Here's how the part is built. I have some questions about the finished solid (model axes, mm). A direction names the side the tool comes from. Give positions to 0.01 mm unless a question says otherwise; leave off trailing zeros. Write each loop counter-clockwise with the first axis right and the second up, starting at its lowest first coordinate (ties: lowest second). Pieces come first, ordered by that corner, then holes. Notation, with made-up numbers: (6, 82) - (64, 82) arc R9 cw to (64, 93) - close; hole circle Ø6 at (-13.75, 88). An arc over 180 degrees is marked (long way). Write each question's results on one line, items separated by ' | '. Start each with the question number.
Item 1: Please list where these lines run through material, in increasing order: line 1 along X through (y, z) = (1.5, 12); line 2 along Y through (x, z) = (2, 0); line 3 along Z through (x, y) = (34, 11.25).
Item 2: Suppose I cut it at B-B on z = 27. List the corners of the cut face in (x, y) for me.
Item 3: Suppose I cut it at A-A on y = 8.55. List the corners of the cut face in (x, z) for me, then the cut area to 3 significant figures.
Item 4: Suppose I cut it at C-C on x = -0.5. List the corners of the cut face in (y, z) for me, then the cut area to 3 significant figures.
Item 5: We'd pull the mould along X, two halves only. Please class faces 1 (the flat face through (20, 8, 33.821)), 2 (the cylindrical face through (31.889, 17.646, 28.891)), 3 (the cylindrical face through (33.25, 10.43, 28.89)): +X half, -X half, draft (parallel to the pull), parting line (faces both ways), or undercut.
Item 6: Which directions (+Z, -Z, +X, -X, +Y, -Y) give clear straight access to the entire face, cutting with the end or side of a thin tool? Please do faces 4 (the flat face through (19.209, 1, 10)), 5 (the cylindrical face through (16.13, 4.3, 28.89)), 6 (the flat face through (9, 1, -4.379)), 7 (the flat face through (7, 3, 14)), 8 (the flat face through (-3.991, 1, 15)).
Item 7: Suppose I cut it at D-D on x = 16. List the corners of the cut face in (y, z) for me.
Item 8: Will these pins go through, and if not, where does the flat tip stop? P1, Ø3.5, axis at x = 6.21, z = 29.82, coming from the +Y side; P2, Ø8, axis at y = 3.5, z = 0.5, coming from the +X side.
```python
from build123d import *

# Parameters (mm, degrees)
SKETCH1_W           = 23.2
SKETCH1_H           = 38.2
SKETCH1_R           = 1.6
BOSS_EXTRUDE1_DEPTH = 3
FILLET1_R           = 4
SKETCH2_R           = 6.25
BOSS_EXTRUDE2_DEPTH = 10
FILLET2_R           = 4


with BuildPart() as part:
    # Sketch1 → Boss-Extrude1 (new body)
    with BuildSketch(Plane(origin=(0, 0, 0), x_dir=(1, 0, 0), z_dir=(0, 1, 0))):
        with Locations((7.60855083, -14.720520933)):
            Rectangle(SKETCH1_W, SKETCH1_H)
        with Locations((0.00855083, 0.379479067)):
            Circle(SKETCH1_R, mode=Mode.SUBTRACT)
        with Locations((6.20855083, -29.820520933)):
            Circle(SKETCH1_R, mode=Mode.SUBTRACT)
    extrude(amount=BOSS_EXTRUDE1_DEPTH)

    # Fillet1
    fillet1_edges = [part.edges().sort_by_distance(p)[0] for p in [
        (-3.99144917, 1.5, -4.379479067),
        (-3.99144917, 1.5, 33.820520933),
    ]]
    fillet(fillet1_edges, radius=FILLET1_R)

    # Sketch2 → Boss-Extrude2 (add)
    with BuildSketch(Plane.XY.offset(33.820520933)):
        with BuildLine():
            Line((19.20855083, 0), (32.911096752, 0.047304531))
            ThreePointArc((32.911096752, 0.047304531), (28.967391183, 18.604369594), (19.20855083, 2.335303477))
            Line((19.20855083, 2.335303477), (19.20855083, 0))
        make_face()
        with Locations((27.28855083, 8.55)):
            Circle(SKETCH2_R, mode=Mode.SUBTRACT)
    extrude(amount=-BOSS_EXTRUDE2_DEPTH)

    # Fillet2
    fillet2_edges = [part.edges().sort_by_distance(p)[0] for p in [
        (18.738325519, 3, 28.820520933),
    ]]
    fillet(fillet2_edges, radius=FILLET2_R)


solid = part.part
```
Checked values:
1) line 1: x = -3.99 to 19.21 | line 2: y = 0 to 3 | line 3: z = 23.82 to 33.82
2) outline: (-3.99, 0) - (19.21, 0) - (32.91, 0.05) arc R10.19 ccw (long way) to (17.16, 7.44) arc R4 cw to (13.18, 3) - (-3.99, 3) - close; hole circle Ø12.5 at (27.29, 8.55)
3) outline: (17.09, 23.82) - (21.04, 23.82) - (21.04, 33.82) - (17.09, 33.82) - close; (33.54, 23.82) - (37.48, 23.82) - (37.48, 33.82) - (33.54, 33.82) - close | area: 78.9 mm^2
4) outline: (0, -4.35) - (3, -4.35) - (3, -1.9) - (0, -1.9) - close; (0, 1.14) - (3, 1.14) - (3, 33.79) - (0, 33.79) - close | area: 105 mm^2
5) face 1: draft | face 2: parting line | face 3: undercut
6) face 4: -Z, +X, +Y, -Y | face 5: +Z, -Z, -X | face 6: -Z, +X, -X, +Y, -Y | face 7: -Z, -X, +Y | face 8: +Z, -Z, -X, +Y, -Y
7) outline: (0, -4.38) - (3, -4.38) - (3, 23.82) - (4.16, 23.82) - (4.16, 33.82) - (0, 33.82) - close
8) P1: stops at y = 3 | P2: stops at x = 19.21
